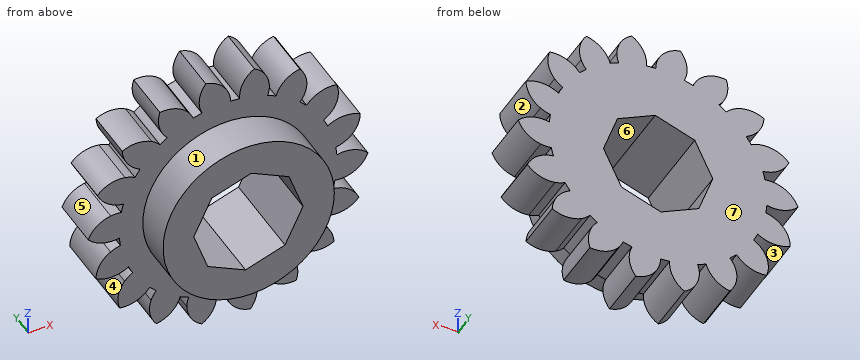
```python
from build123d import *

# Parameters (mm, degrees)
F0_R     = 42.21774
F1_DEPTH = 25.4
F2_COUNT = 18
F3_DEPTH = 45


with BuildPart() as f1:
    # F0 (on Front) → F1 (new body)
    with BuildSketch(Plane.XZ):
        with BuildLine():
            ThreePointArc((-12.918881, 52.144495), (-33.105367, -42.308161), (53.721, 0))
            ThreePointArc((53.721, 0), (38.40509, 37.563212), (1.190523, 53.707807))
            ThreePointArc((1.190523, 53.707807), (-5.916044, 53.394253), (-12.918881, 52.144495))
        make_face()
        with Locations((0.154254, 0.462766)):
            Circle(F0_R, mode=Mode.SUBTRACT)
        with BuildLine():
            ThreePointArc((-12.918881, 52.144495), (-5.916044, 53.394253), (1.190523, 53.707807))
            ThreePointArc((1.190523, 53.707807), (0.942954, 56.310266), (0.237615, 58.827522))
            ThreePointArc((0.237615, 58.827522), (-4.155035, 64.953488), (-11.009105, 68.091091))
            ThreePointArc((-11.009105, 68.091091), (-14.1755, 60.382645), (-12.918881, 52.144495))
        make_face()
    extrude(amount=F1_DEPTH)

    # F2: F1 ×18 about axis
    f2_axis = Axis((0, 0, 0), (0, 1, 0))


with BuildPart() as f1_1:
    add(f1.part)
    for i in range(1, F2_COUNT):
        add(f1.part.rotate(f2_axis, i * 360 / F2_COUNT))

    # F0 (on Front) → F3 (join)
    with BuildSketch(Plane.XZ):
        with Locations((0.154254, 0.462766)):
            Circle(F0_R)
        Polygon((-26.953759, 1.414539), (-18.058955, 20.059416), (1.414539, 26.953759), (20.059416, 18.058955), (26.953759, -1.414539), (18.058955, -20.059416), (-1.414539, -26.953759), (-20.059416, -18.058955), align=None, mode=Mode.SUBTRACT)
    extrude(amount=F3_DEPTH)


solid = f1_1.part
```
For this review, take the finished solid that the model builds, in its own axes (mm). Face numbers are marked on the shaded views. A direction names the side the tool comes from. Round coordinates to 2 decimals unless told otherwise and drop trailing zeros. Loops run counter-clockwise (first coordinate to the right, second up) from the corner with the lowest first, then second, coordinate; pieces in that order, holes last.
(1) We need section A-A (y = -36). Give the boundary of the cut face in (x, z).
Returned:
outline: circle Ø84.44 at (0.15, 0.46); hole (-26.95, 1.41) - (-20.06, -18.06) - (-1.41, -26.95) - (18.06, -20.06) - (26.95, -1.41) - (20.06, 18.06) - (1.41, 26.95) - (-18.06, 20.06) - close
(2) Wall thickness on line 1 along X through (y, z) = (-18, 55); line 2 along Z through (x, y) = (-62, -20.5); line 3 along Y through (x, z) = (0.5, 56.5): over which ranges is each line inside the solid? List them lowest first.
Returned:
line 1: x = -34.38 to -19.6, -13.88 to 1.13, 5.66 to 20.34, 27.58 to 37.84
line 2: z = -23.91 to -13.51, -3.45 to 9.01, 20.4 to 26.87
line 3: y = -25.4 to 0
(3) Mouldability with a two-part tool opening along X and no side actions: class the marked faces 1, 2, 3 and 4 as released by +X, released by -X, zero draft, split by the parting line, or undercut.
Returned:
face 1: split by the parting line
face 2: released by +X
face 3: undercut
face 4: released by -X
(4) Clearance check with flat-ended pins moving along their axes: P1, Ø1.5, axis at x = -40, z = 17, coming from the -Y side; P2, Ø1, axis at x = 18, y = -10.5, coming from the +Z side; P3, Ø8, axis at x = -14.5, y = -13, coming from the -Z side. State where each tip first meets the part, or that it passes through.
Returned:
P1: stops at y = -25.4
P2: stops at z = 63.69
P3: stops at z = -67.75
(5) We need section B-B (x = -56). Give the boundary of the cut face in (y, z).
Returned:
outline: (-25.4, -24.36) - (0, -24.36) - (0, -9) - (-25.4, -9) - close; (-25.4, -4.08) - (0, -4.08) - (0, 10.68) - (-25.4, 10.68) - close; (-25.4, 15.99) - (0, 15.99) - (0, 29.54) - (-25.4, 29.54) - close
(6) Tool access review of the marked faces 5, 6 and 7: name each direction out of +Z, -Z, +X, -X, +Y, -Y from which nothing blocks a thin tool from reaching the whole face with its end or side.
Returned:
face 5: -X, +Y, -Y
face 6: +Y, -Y
face 7: +Z, -Z, +X, -X, +Y
